Source: CAD feature listing. Evaluate the final solid. Frame: model axes, mm. Give positions to 0.01 mm unless a question says otherwise; leave off trailing zeros. Order: outer loops, then holes, each group sorted by start corner. A loop starts at its lowest first (then second) coordinate and runs counter-clockwise, first axis right, second up.
1) Section B-B, the plane z = 0. Return loops of the section in (x, y), plus the area to 3 significant figures.
2) Section C-C, the plane x = -66. Return loops of the section in (y, z), plus the area to 3 significant figures.
3) Section A-A, the plane x = 0. Return loops of the section in (y, z).
4) Section D-D, the plane z = -30. Return loops of the section in (x, y), plus the area to 3 significant figures.
5) First-contact query: P1, Ø3, axis at x = -30.62, z = -50.84, coming from the -Y side; P2, Ø2, axis at y = -1, z = 59.5, coming from the +X side; P3, Ø1, axis at x = -7, y = -2, coming from the +Z side; P4, Ø3, axis at y = -3, z = 49.5, coming from the -X side. Flat tips, straight axial feed; report the tip coordinate or a pass-through.
6) Material intervals for line 1 (Z direction, x = -61, y = -3.5); line 2 (Z direction, x = 52.5, y = -0.9); line 3 (Z direction, x = 46, y = -3.6), sorted ascending.
```python
from build123d import *

# Parameters (mm, degrees)
SKETCH2_R           = 15
SKETCH2_R_2         = 5
SKETCH2_R_3         = 2.5
BOSS_EXTRUDE1_DEPTH = 5


with BuildPart() as part:
    # Sketch2 → Boss-Extrude1 (new body)
    with BuildSketch(Plane(origin=(0, 0, 0), x_dir=(1, 0, 0), z_dir=(0, 1, 0))):
        with BuildLine():
            Line((45, 75), (75, 45))
            ThreePointArc((75, 45), (56.360389693, 0), (75, -45))
            Line((75, -45), (45, -75))
            ThreePointArc((45, -75), (0, -56.360389693), (-45, -75))
            Line((-45, -75), (-75, -45))
            ThreePointArc((-75, -45), (-56.360389693, 0), (-75, 45))
            Line((-75, 45), (-45, 75))
            ThreePointArc((-45, 75), (0, 56.360389693), (45, 75))
        make_face()
        with Locations(Location((0, 0, 0), (0, 0, 270))):
            Circle(SKETCH2_R, mode=Mode.SUBTRACT)
        with Locations(Location((30, 30, 0), (0, 0, 270))):
            Circle(SKETCH2_R_2, mode=Mode.SUBTRACT)
        with Locations(Location((42.426406871, 0, 0), (0, 0, 270))):
            Circle(SKETCH2_R_2, mode=Mode.SUBTRACT)
        with Locations(Location((30, -30, 0), (0, 0, 270))):
            Circle(SKETCH2_R_2, mode=Mode.SUBTRACT)
        with Locations(Location((0, -42.426406871, 0), (0, 0, 270))):
            Circle(SKETCH2_R_2, mode=Mode.SUBTRACT)
        with Locations(Location((-30, -30, 0), (0, 0, 270))):
            Circle(SKETCH2_R_2, mode=Mode.SUBTRACT)
        with Locations(Location((-42.426406871, 0, 0), (0, 0, 270))):
            Circle(SKETCH2_R_2, mode=Mode.SUBTRACT)
        with Locations(Location((-30, 30, 0), (0, 0, 270))):
            Circle(SKETCH2_R_2, mode=Mode.SUBTRACT)
        with Locations(Location((0, 42.426406871, 0), (0, 0, 270))):
            Circle(SKETCH2_R_2, mode=Mode.SUBTRACT)
        with Locations(Location((41.228106405, 61.448235065, 0), (0, 0, 270))):
            Circle(SKETCH2_R_3, mode=Mode.SUBTRACT)
        with Locations(Location((30.621504688, 50.841633347, 0), (0, 0, 270))):
            Circle(SKETCH2_R_3, mode=Mode.SUBTRACT)
        with Locations(Location((61.448235065, 41.228106405, 0), (0, 0, 90))):
            Circle(SKETCH2_R_3, mode=Mode.SUBTRACT)
        with Locations(Location((50.841633347, 30.621504688, 0), (0, 0, 90))):
            Circle(SKETCH2_R_3, mode=Mode.SUBTRACT)
        with Locations(Location((61.448235065, -41.228106405, 0), (0, 0, 270))):
            Circle(SKETCH2_R_3, mode=Mode.SUBTRACT)
        with Locations(Location((50.841633347, -30.621504688, 0), (0, 0, 270))):
            Circle(SKETCH2_R_3, mode=Mode.SUBTRACT)
        with Locations(Location((41.228106405, -61.448235065, 0), (0, 0, 90))):
            Circle(SKETCH2_R_3, mode=Mode.SUBTRACT)
        with Locations(Location((30.621504688, -50.841633347, 0), (0, 0, 90))):
            Circle(SKETCH2_R_3, mode=Mode.SUBTRACT)
        with Locations(Location((-41.228106405, -61.448235065, 0), (0, 0, 270))):
            Circle(SKETCH2_R_3, mode=Mode.SUBTRACT)
        with Locations(Location((-30.621504688, -50.841633347, 0), (0, 0, 270))):
            Circle(SKETCH2_R_3, mode=Mode.SUBTRACT)
        with Locations(Location((-61.448235065, -41.228106405, 0), (0, 0, 90))):
            Circle(SKETCH2_R_3, mode=Mode.SUBTRACT)
        with Locations(Location((-50.841633347, -30.621504688, 0), (0, 0, 90))):
            Circle(SKETCH2_R_3, mode=Mode.SUBTRACT)
        with Locations(Location((-61.448235065, 41.228106405, 0), (0, 0, 270))):
            Circle(SKETCH2_R_3, mode=Mode.SUBTRACT)
        with Locations(Location((-50.841633347, 30.621504688, 0), (0, 0, 270))):
            Circle(SKETCH2_R_3, mode=Mode.SUBTRACT)
        with Locations(Location((-41.228106405, 61.448235065, 0), (0, 0, 90))):
            Circle(SKETCH2_R_3, mode=Mode.SUBTRACT)
        with Locations(Location((-30.621504688, 50.841633347, 0), (0, 0, 90))):
            Circle(SKETCH2_R_3, mode=Mode.SUBTRACT)
        with BuildLine():
            Line((38.610248674, 42.852889361), (42.852889361, 38.610248674))
            ThreePointArc((42.852889361, 38.610248674), (44.267102923, 38.024462236), (45.681316486, 38.610248674))
            Line((45.681316486, 38.610248674), (56.995024985, 49.923957173))
            ThreePointArc((56.995024985, 49.923957173), (57.580811422, 51.338170735), (56.995024985, 52.752384297))
            Line((56.995024985, 52.752384297), (52.752384297, 56.995024985))
            ThreePointArc((52.752384297, 56.995024985), (51.338170735, 57.580811422), (49.923957173, 56.995024985))
            Line((49.923957173, 56.995024985), (38.610248674, 45.681316486))
            ThreePointArc((38.610248674, 45.681316486), (38.024462236, 44.267102923), (38.610248674, 42.852889361))
        make_face(mode=Mode.SUBTRACT)
        with BuildLine():
            Line((45.681316486, -38.610248674), (56.995024985, -49.923957173))
            ThreePointArc((56.995024985, -49.923957173), (57.580811422, -51.338170735), (56.995024985, -52.752384297))
            Line((56.995024985, -52.752384297), (52.752384297, -56.995024985))
            ThreePointArc((52.752384297, -56.995024985), (51.338170735, -57.580811422), (49.923957173, -56.995024985))
            Line((49.923957173, -56.995024985), (38.610248674, -45.681316486))
            ThreePointArc((38.610248674, -45.681316486), (38.024462236, -44.267102923), (38.610248674, -42.852889361))
            Line((38.610248674, -42.852889361), (42.852889361, -38.610248674))
            ThreePointArc((42.852889361, -38.610248674), (44.267102923, -38.024462236), (45.681316486, -38.610248674))
        make_face(mode=Mode.SUBTRACT)
        with BuildLine():
            Line((-38.610248674, -45.681316486), (-49.923957173, -56.995024985))
            ThreePointArc((-49.923957173, -56.995024985), (-51.338170735, -57.580811422), (-52.752384297, -56.995024985))
            Line((-52.752384297, -56.995024985), (-56.995024985, -52.752384297))
            ThreePointArc((-56.995024985, -52.752384297), (-57.580811422, -51.338170735), (-56.995024985, -49.923957173))
            Line((-56.995024985, -49.923957173), (-45.681316486, -38.610248674))
            ThreePointArc((-45.681316486, -38.610248674), (-44.267102923, -38.024462236), (-42.852889361, -38.610248674))
            Line((-42.852889361, -38.610248674), (-38.610248674, -42.852889361))
            ThreePointArc((-38.610248674, -42.852889361), (-38.024462236, -44.267102923), (-38.610248674, -45.681316486))
        make_face(mode=Mode.SUBTRACT)
        with BuildLine():
            Line((-45.681316486, 38.610248674), (-56.995024985, 49.923957173))
            ThreePointArc((-56.995024985, 49.923957173), (-57.580811422, 51.338170735), (-56.995024985, 52.752384297))
            Line((-56.995024985, 52.752384297), (-52.752384297, 56.995024985))
            ThreePointArc((-52.752384297, 56.995024985), (-51.338170735, 57.580811422), (-49.923957173, 56.995024985))
            Line((-49.923957173, 56.995024985), (-38.610248674, 45.681316486))
            ThreePointArc((-38.610248674, 45.681316486), (-38.024462236, 44.267102923), (-38.610248674, 42.852889361))
            Line((-38.610248674, 42.852889361), (-42.852889361, 38.610248674))
            ThreePointArc((-42.852889361, 38.610248674), (-44.267102923, 38.024462236), (-45.681316486, 38.610248674))
        make_face(mode=Mode.SUBTRACT)
    extrude(amount=-BOSS_EXTRUDE1_DEPTH)


solid = part.part
```
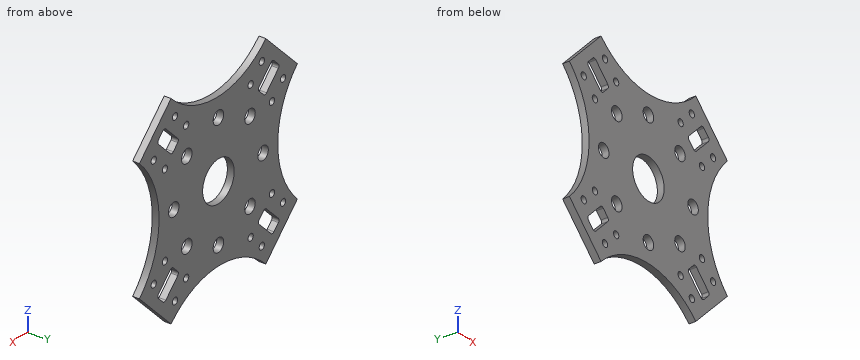
From the geometry:
1. outline: (-56.36, -5) - (-47.43, -5) - (-47.43, 0) - (-56.36, 0) - close; (-37.43, -5) - (-15, -5) - (-15, 0) - (-37.43, 0) - close; (15, -5) - (37.43, -5) - (37.43, 0) - (15, 0) - close; (47.43, -5) - (56.36, -5) - (56.36, 0) - (47.43, 0) - close
1. area: 314 mm2
2. outline: (-5, -54) - (0, -54) - (0, -33.67) - (-5, -33.67) - close; (-5, 33.67) - (0, 33.67) - (0, 54) - (-5, 54) - close
2. area: 203 mm2
3. outline: (-5, -56.36) - (0, -56.36) - (0, -47.43) - (-5, -47.43) - close; (-5, -37.43) - (0, -37.43) - (0, -15) - (-5, -15) - close; (-5, 15) - (0, 15) - (0, 37.43) - (-5, 37.43) - close; (-5, 47.43) - (0, 47.43) - (0, 56.36) - (-5, 56.36) - close
4. outline: (-63.88, -5) - (-53.26, -5) - (-53.26, 0) - (-63.88, 0) - close; (-48.42, -5) - (-35, -5) - (-35, 0) - (-48.42, 0) - close; (-25, -5) - (25, -5) - (25, 0) - (-25, 0) - close; (35, -5) - (48.42, -5) - (48.42, 0) - (35, 0) - close; (53.26, -5) - (63.88, -5) - (63.88, 0) - (53.26, 0) - close
4. area: 490 mm2
5. P1: passes through
5. P2: stops at x = 61.5
5. P3: stops at z = 56.8
5. P4: stops at x = -72
6. line 1: z = -59 to -43.69, -38.77 to -23.85, 23.85 to 38.77, 43.69 to 59
6. line 2: z = -67.5 to -57.21, -45.43 to -32.49, -28.75 to 28.75, 32.49 to 45.43, 57.21 to 67.5
6. line 3: z = -74 to -53.07, -38.93 to -3.5, 3.5 to 38.93, 53.07 to 74
